For this review, use the dimensioned drawing (mm, ordinates from the lowest corner) and the shaded views. A direction names the side the tool comes from. Round coordinates to 2 decimals unless told otherwise and drop trailing zeros. Write each loop counter-clockwise with the first axis right and the second up, starting at its lowest first coordinate (ties: lowest second). Pieces come first, ordered by that corner, then holes. Notation, with made-up numbers: M 12,76 L 40,76 A30 ccw 40,98 Z; hole C 60,66 d3. An arc over 180 degrees is marked long. Use CSV: the item, a comma, the result in double quotes.
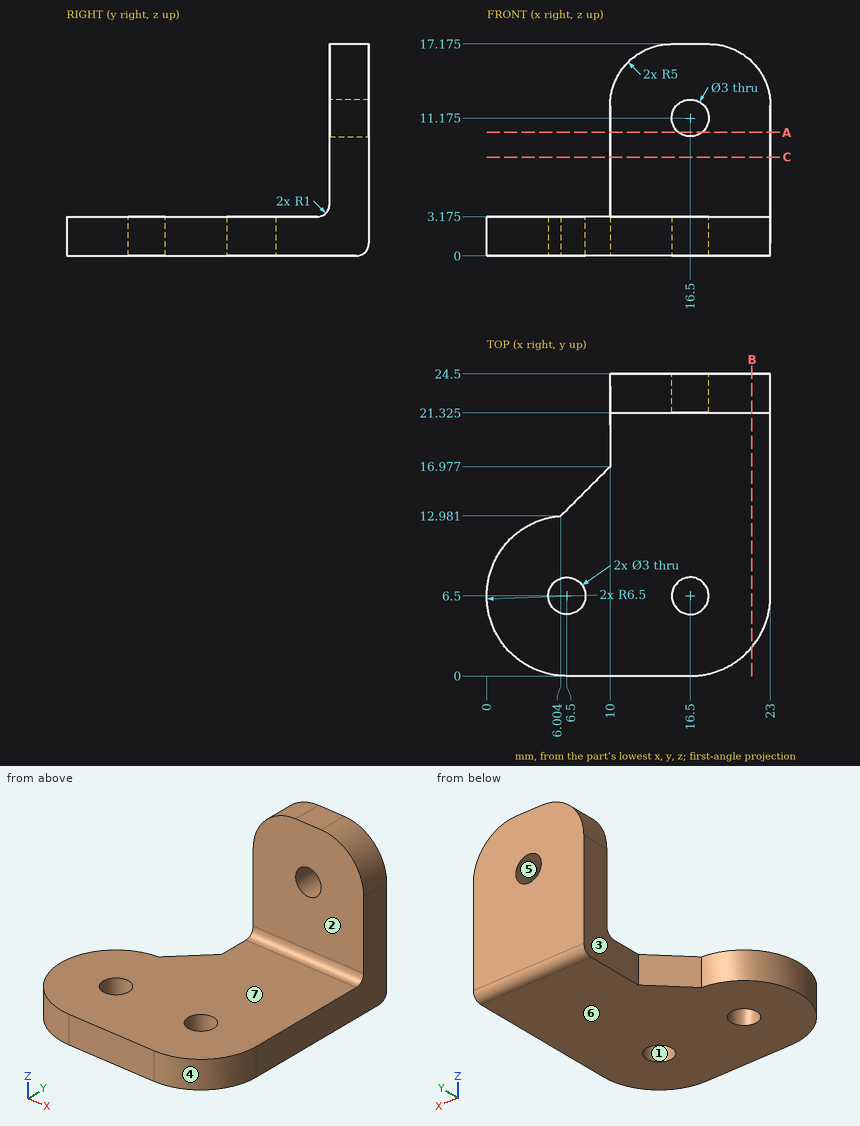
1) The part is to be moulded in two halves that separate along Z. For the marked faces 4, 5, 6 and 7, say which applies: released by +Z, released by -Z, zero draft, split by the parting line, or undercut.
Answers:
face 4,"zero draft"
face 5,"undercut"
face 6,"released by -Z"
face 7,"released by +Z"
2) Machinability: for the marked faces 1, 2 and 3, which of the approach directions +Z, -Z, +X, -X, +Y, -Y give a long, thin tool a straight path to every point of the face, cutting with its end or side? Answer none if there is none.
Answers:
face 1,"+Z, -Z"
face 2,"+Z, +X, -X, -Y"
face 3,"+Z, -Z, -X, +Y"
3) Add section C-C on z = 8. Write out the cut boundary in (x, y) (3 decimals).
Answers:
outline,"M 10,21.325 L 23,21.325 L 23,24.5 L 10,24.5 Z"
4) For pin 1 Ø8.5 at (y, z) = (20.5, 4.5) entering from -X (1 decimal); pin 2 Ø6 at (x, z) = (9, 10.5) entering from -Y (3 decimals); pin 3 Ø10 at (x, y) = (11.5, 10) entering from +Z (3 decimals), all flat-tipped, find the tip position at first contact; note any pin that passes through.
Answers:
pin 1,"x = 9.5"
pin 2,"y = 21.325"
pin 3,"z = 3.175"
5) Add section A-A on z = 10. Write out the cut boundary in (x, y) (1 decimal).
Answers:
outline,"M 10,21.3 L 15.6,21.3 L 15.6,24.5 L 10,24.5 Z; M 17.4,21.3 L 23,21.3 L 23,24.5 L 17.4,24.5 Z"
6) Add section B-B on x = 21.5. Write out the cut boundary in (y, z) (1 decimal), then the cut area to 3 significant figures.
Answers:
outline,"M 2.3,0 L 23.5,0 A1 ccw 24.5,1 L 24.5,15.7 L 21.3,15.7 L 21.3,4.2 A1 cw 20.3,3.2 L 2.3,3.2 Z"
area,"110 mm²"
7) Wall thickness on line 1 along Z through (x, y) = (21.5, 16) (3 decimals); line 2 along X through (y, z) = (23.75, 8.25); line 3 along Y through (x, z) = (22, 12.5) (3 decimals): over which ranges is each line inside the solid? List them lowest first. Write a range as [from, to].
Answers:
line 1,"[0, 3.175]"
line 2,"[10, 23]"
line 3,"[21.325, 24.5]"
